Design review of the part built by this model. Coordinates are the model's own, in mm. A direction names the side the tool comes from. Round coordinates to 2 decimals unless told otherwise and drop trailing zeros. Order: outer loops, then holes, each group sorted by start corner. A loop starts at its lowest first (then second) coordinate and runs counter-clockwise, first axis right, second up.
from build123d import *

# Parameters (mm, degrees)
SKETCH1_R             = 10
BOSS_EXTRUDE2_DEPTH   = 7
BOSS_EXTRUDE2_2_DEPTH = 7
BOSS_EXTRUDE3_DEPTH   = 17
CUT_EXTRUDE1_START    = -10
CUT_EXTRUDE1_DEPTH    = 10
CUT_EXTRUDE2_DEPTH    = 113.649900133
SKETCH5_R             = 7
CUT_EXTRUDE3_DEPTH    = 5
SKETCH6_W             = 80
SKETCH6_H             = 34
CUT_EXTRUDE4_DEPTH    = 113.649900133
SKETCH7_W             = 80
SKETCH7_H             = 34
SKETCH7_W_2           = 74
SKETCH7_H_2           = 28
BOSS_EXTRUDE4_DEPTH   = 10
CUT_EXTRUDE5_DEPTH    = 113.649900133
SKETCH9_W             = 90
SKETCH9_H             = 5
BOSS_EXTRUDE5_DEPTH   = 8.75
SKETCH10_W            = 16
SKETCH10_H            = 3
BOSS_EXTRUDE6_DEPTH   = 8.717948718
CUT_EXTRUDE6_DEPTH    = 11


with BuildPart() as part:
    # Sketch1 → Boss-Extrude2 (new body)
    with BuildSketch(Plane(origin=(0, 0, 0), x_dir=(0, 0, -1), z_dir=(1, 0, 0))):
        Circle(SKETCH1_R)
    extrude(amount=BOSS_EXTRUDE2_DEPTH)



with BuildPart() as body_2:
    # Sketch1 → Boss-Extrude2 2 (new body)
    with BuildSketch(Plane(origin=(0, 0, 0), x_dir=(0, 0, -1), z_dir=(1, 0, 0))):
        with Locations((90, 0)):
            Circle(SKETCH1_R)
    extrude(amount=BOSS_EXTRUDE2_2_DEPTH)


with BuildPart() as part_1:
    add(part.part)

    add(body_2.part)  # Boss-Extrude3 merges body 2
    # Sketch1<3> → Boss-Extrude3 (add)
    with BuildSketch(Plane(origin=(0, 0, 0), x_dir=(0, 0, -1), z_dir=(1, 0, 0))):
        with BuildLine():
            Line((80, 0), (10, 0))
            ThreePointArc((10, 0), (7.071067812, -7.071067812), (0, -10))
            Line((0, -10), (0, -49))
            Line((0, -49), (90, -49))
            Line((90, -49), (90, -10))
            ThreePointArc((90, -10), (82.928932188, -7.071067812), (80, 0))
        make_face()
    extrude(amount=BOSS_EXTRUDE3_DEPTH)

    # Sketch3 → Cut-Extrude1 (cut)
    with BuildSketch(Plane(origin=(17, 0, 0), x_dir=(0, 0, -1), z_dir=(1, 0, 0)).offset(CUT_EXTRUDE1_START)):
        with BuildLine():
            Line((0, -10), (90, -10))
            ThreePointArc((90, -10), (82.928932188, -7.071067812), (80, 0))
            Line((80, 0), (10, 0))
            ThreePointArc((10, 0), (7.071067812, -7.071067812), (0, -10))
        make_face()
    extrude(amount=CUT_EXTRUDE1_DEPTH, mode=Mode.SUBTRACT)

    # Sketch4 → Cut-Extrude2 (cut, through all)
    with BuildSketch(Plane.XY):
        Polygon((7, -10), (17, -49), (17, -10), align=None)
    extrude(amount=-CUT_EXTRUDE2_DEPTH, mode=Mode.SUBTRACT)

    # Sketch5 → Cut-Extrude3 (cut)
    with BuildSketch(Plane(origin=(7, 0, 0), x_dir=(0, 0, -1), z_dir=(1, 0, 0))):
        Circle(SKETCH5_R)
        with Locations((90, 0)):
            Circle(SKETCH5_R)
    extrude(amount=-CUT_EXTRUDE3_DEPTH, mode=Mode.SUBTRACT)

    # Sketch6 → Cut-Extrude4 (cut, through all)
    with BuildSketch(Plane.ZY):
        with Locations((-45, -27)):
            Rectangle(SKETCH6_W, SKETCH6_H)
    extrude(amount=-CUT_EXTRUDE4_DEPTH, mode=Mode.SUBTRACT)

    # Sketch7 → Boss-Extrude4 (add)
    with BuildSketch(Plane.ZY):
        with Locations((-45, -27)):
            Rectangle(SKETCH7_W, SKETCH7_H)
        with Locations((-45, -27)):
            Rectangle(SKETCH7_W_2, SKETCH7_H_2, mode=Mode.SUBTRACT)
    extrude(amount=-BOSS_EXTRUDE4_DEPTH)

    # Sketch8 → Cut-Extrude5 (cut, through all)
    with BuildSketch(Plane.XY):
        Polygon((15.717948718, -44), (17, -49), (6.967948718, -49), (6.967948718, -44), align=None)
    extrude(amount=-CUT_EXTRUDE5_DEPTH, mode=Mode.SUBTRACT)

    # Sketch9 → Boss-Extrude5 (add)
    with BuildSketch(Plane(origin=(6.967948718, 0, 0), x_dir=(0, 0, -1), z_dir=(1, 0, 0))):
        with Locations((45, -46.5)):
            Rectangle(SKETCH9_W, SKETCH9_H)
    extrude(amount=BOSS_EXTRUDE5_DEPTH)

    # Sketch10 → Boss-Extrude6 (add)
    with BuildSketch(Plane(origin=(15.717948718, 0, 0), x_dir=(0, 0, -1), z_dir=(1, 0, 0))):
        with Locations((45, -42.5)):
            Rectangle(SKETCH10_W, SKETCH10_H)
    extrude(amount=-BOSS_EXTRUDE6_DEPTH)

    # Sketch11 → Cut-Extrude6 (cut)
    with BuildSketch(Plane(origin=(0, -41, 0), x_dir=(1, 0, 0), z_dir=(0, 1, 0))):
        with BuildLine():
            Line((15.717948718, 42), (8.717948718, 42))
            ThreePointArc((8.717948718, 42), (5.717948718, 45), (8.717948718, 48))
            Line((8.717948718, 48), (15.717948718, 48))
            Line((15.717948718, 48), (15.717948718, 42))
        make_face()
    extrude(amount=-CUT_EXTRUDE6_DEPTH, mode=Mode.SUBTRACT)


solid = part_1.part
1) Clearance check with flat-ended pins moving along their axes: P1, Ø1.5, axis at x = 8.5, y = -18.5, coming from the +Z side; P2, Ø6, axis at x = 14, z = -15.5, coming from the +Y side; P3, Ø5.5, axis at x = 3.5, z = -44.5, coming from the +Y side. State where each tip first meets the part, or that it passes through.
Results:
P1: stops at z = 0
P2: stops at y = -44
P3: stops at y = 0
2) For faces 1 (the face through (9, -13, -85)), 2 (the face through (5, -13, -46)), 3 (the face through (13, -44, -21)), 4 (the face through (7, -4, -44)), 5 (the face through (12, -45, -48)), list the 3-axis set-ups (+Z, -Z, +X, -X, +Y, -Y) from which the entire face can be reached by the end or side of a thin tool; tool diameter is ignored.
Results:
face 1: -Z, +X, +Y
face 2: +X, -X
face 3: +X, +Y
face 4: +Z, -Z, +X, +Y
face 5: +X, -Y
3) Take a section at A-A on z = -50. Give the boundary of the cut face in (x, y).
Results:
outline: (0, -49) - (15.72, -49) - (15.72, -41) - (0, -41) - close; (0, -13) - (10, -13) - (10, -10) - (7, -10) - (7, 0) - (0, 0) - close
4) The part is to be moulded in two halves that separate along Y. For faces 6 (the face through (12, -35, -5)), 7 (the face through (3.451, 6.834, -97.3)), 8 (the face through (5, -27, -8)), say which applies: released by +Y, released by -Y, zero draft, split by the parting line, or undercut.
Results:
face 6: zero draft
face 7: split by the parting line
face 8: undercut
5) Take a section at C-C on y = -39.5. Give the boundary of the cut face in (x, z), plus the area to 3 significant figures.
Results:
outline: (0, -90) - (14.56, -90) - (14.56, -85) - (10, -85) - (10, -82) - (0, -82) - close; (0, -8) - (10, -8) - (10, -5) - (14.56, -5) - (14.56, 0) - (0, 0) - close
area: 206 mm2
6) Take a section at B-B on y = 3.5. Give the boundary of the cut face in (x, z).
Results:
outline: (0, -99.37) - (7, -99.37) - (7, -96.06) - (2, -96.06) - (2, -83.94) - (7, -83.94) - (7, -80.63) - (0, -80.63) - close; (0, -9.37) - (7, -9.37) - (7, -6.06) - (2, -6.06) - (2, 6.06) - (7, 6.06) - (7, 9.37) - (0, 9.37) - close
7) To check wall thickness, follow line 1 along Y through (x, z) = (4, -26.5); line 2 along Z through (x, y) = (9.25, -29); line 3 along Y through (x, z) = (14, -59.5). State the ranges of each line that lie inside material, in increasing order.
Results:
line 1: y = -49 to -41, -13 to 0
line 2: z = -90 to -82, -8 to 0
line 3: y = -49 to -44
8) Take a section at D-D on y = -3. Give the boundary of the cut face in (x, z), plus the area to 3 significant figures.
Results:
outline: (0, -99.54) - (7, -99.54) - (7, -96.32) - (2, -96.32) - (2, -83.68) - (7, -83.68) - (7, -6.32) - (2, -6.32) - (2, 6.32) - (7, 6.32) - (7, 9.54) - (0, 9.54) - close
area: 637 mm2
